Verification items for the finished model (mm, model axes). Face numbers are marked on the shaded views. A direction names the side the tool comes from. Coordinates: 2 decimals unless noted, no trailing zeros. Order: outer loops, then holes, each group sorted by start corner. A loop starts at its lowest first (then second) coordinate and runs counter-clockwise, first axis right, second up. Notation, with made-up numbers: (-12.5, 21) - (3.5, 21) arc R16 cw to (3.5, 52) - close; hole circle Ø11 at (26.5, 64.5). An arc over 180 degrees is marked (long way). One line per question, with ' | ' between items. Start each with the question number.
from build123d import *

# Parameters (mm, degrees)
SKETCH_1_W                = 48.51
SKETCH_1_H                = 34
SKETCH_1_W_2              = 28.51
SKETCH_1_H_2              = 14
EXTRUDE_1_DEPTH           = 12.25
SKETCH_2_R                = 1.91
CUT_EXTRUDE_1_DEPTH       = 33.05257439
SKETCH_4_W                = 13
SKETCH_4_H                = 13.91
EXTRUDE_1_2_DEPTH         = 74.82
SKETCH_5_W                = 13.91
SKETCH_5_H                = 16.23
EXTRUDE_2_DEPTH           = 15
SKETCH_7_R                = 24.5
SKETCH_7_R_2              = 14.5
EXTRUDE_2_2_DEPTH         = 16.23
SKETCH_12_R               = 1.9
CUT_EXTRUDE_4_DEPTH       = 97.312124675
EXTRUDE_3_DEPTH           = 10
EXTRUDE_3_DEPTH_BACK      = 8
SKETCH_13_W               = 13.91
SKETCH_13_H               = 16.23
SKETCH_14_R               = 1.9
CUT_EXTRUDE_5_DEPTH       = 103.744583434
SKETCH_16_W               = 90.709398763
SKETCH_16_H               = 28.955068616
CUT_EXTRUDE_7_DEPTH       = 111.229011154
SKETCH_18_W               = 13
SKETCH_18_H               = 93.080932143
CUT_EXTRUDE_10_DEPTH      = 27
CUT_EXTRUDE_11_DEPTH      = 57
CUT_EXTRUDE_11_DEPTH_BACK = 27
SKETCH_17_W               = 20.23049449
SKETCH_17_H               = 80.723570055


with BuildPart() as part:
    # 草圖1 → Extrude 1 (new body)
    with BuildSketch(Plane(origin=(0, 0, 0), x_dir=(1, 0, 0), z_dir=(0, 1, 0))):
        Rectangle(SKETCH_1_W, SKETCH_1_H)
        Rectangle(SKETCH_1_W_2, SKETCH_1_H_2, mode=Mode.SUBTRACT)
    extrude(amount=EXTRUDE_1_DEPTH)

    # 草圖2 → 除料-伸長1 (cut, through all)
    with BuildSketch(Plane(origin=(0, 12.25, 0), x_dir=(1, 0, 0), z_dir=(0, 1, 0))):
        with Locations(Location((-19.255, 0, 0), (0, 0, 270))):
            Circle(SKETCH_2_R)
        with Locations(Location((19.255, 0, 0), (0, 0, 270))):
            Circle(SKETCH_2_R)
    extrude(amount=-CUT_EXTRUDE_1_DEPTH, mode=Mode.SUBTRACT)

    # 草圖4 → Extrude 1 2 (add)
    with BuildSketch(Plane.XZ):
        with Locations((17.755, 0)):
            Rectangle(SKETCH_4_W, SKETCH_4_H)
    extrude(amount=EXTRUDE_1_2_DEPTH)

    # 草圖5 → Extrude 2 (add)
    with BuildSketch(Plane.ZY.offset(-11.255)):
        with Locations((0, -66.705)):
            Rectangle(SKETCH_5_W, SKETCH_5_H)
    extrude(amount=EXTRUDE_2_DEPTH)

    # 草圖7 → Extrude 2 2 (add)
    with BuildSketch(Plane(origin=(3.626674765, -74.82, 0), x_dir=(1, 0, 0), z_dir=(0, -1, 0))):
        with Locations((-30.978154344, 0)):
            Circle(SKETCH_7_R)
        with Locations((-30.978154344, 0)):
            Circle(SKETCH_7_R_2, mode=Mode.SUBTRACT)
    extrude(amount=-EXTRUDE_2_2_DEPTH)

    # 草圖12 → 除料-伸長4 (cut, through all)
    with BuildSketch(Plane(origin=(0, 0, -6.955), x_dir=(-1, 0, 0), z_dir=(0, 0, -1))):
        with Locations((-3.856713649, -66.705)):
            Circle(SKETCH_12_R)
    extrude(amount=-CUT_EXTRUDE_4_DEPTH, mode=Mode.SUBTRACT)

    # 草圖13 → 填料-伸長3 (add, two sides: drawn at the far end of the back side and taken through both)
    with BuildSketch(Plane(origin=(-55, 0, 0), x_dir=(0, 0, -1), z_dir=(1, 0, 0)).offset(-EXTRUDE_3_DEPTH_BACK)):
        with Locations((0, -66.705)):
            Rectangle(SKETCH_13_W, SKETCH_13_H)
    extrude(amount=EXTRUDE_3_DEPTH + EXTRUDE_3_DEPTH_BACK)

    # 草圖14 → 除料-伸長5 (cut, through all)
    with BuildSketch(Plane(origin=(0, 0, -6.955), x_dir=(-1, 0, 0), z_dir=(0, 0, -1))):
        with Locations((56.908040017, -66.705)):
            Circle(SKETCH_14_R)
    extrude(amount=-CUT_EXTRUDE_5_DEPTH, mode=Mode.SUBTRACT)

    # 草圖16 → 除料-伸長7 (cut, through all)
    with BuildSketch(Plane(origin=(0, 12.25, 0), x_dir=(1, 0, 0), z_dir=(0, 1, 0))):
        with Locations((-17.645300619, -14.477534308)):
            Rectangle(SKETCH_16_W, SKETCH_16_H)
    extrude(amount=-CUT_EXTRUDE_7_DEPTH, mode=Mode.SUBTRACT)

    # 草圖18 → 除料-伸長10 (cut)
    with BuildSketch(Plane.XY):
        with Locations((17.755, -28.279533929)):
            Rectangle(SKETCH_18_W, SKETCH_18_H)
    extrude(amount=-CUT_EXTRUDE_10_DEPTH, mode=Mode.SUBTRACT)


with BuildPart() as cut_extrude_10_piece_1:
    # of the separate pieces the step leaves, piece 1, a body of its own (cut_extrude_10_pieces)
    add(part.part.solids().sort_by_distance((11.255, -58.59, -6.955))[0])


with BuildPart() as cut_extrude_10_piece_2:
    # of the separate pieces the step leaves, piece 2, a body of its own (cut_extrude_10_pieces)
    add(part.part.solids().sort_by_distance((-17.345, 0, 0))[0])

    # 草圖17 → 除料-伸長11 (cut, two sides: drawn at the far end of the back side and taken through both)
    with BuildSketch(Plane.ZY.offset(-11.255).offset(-CUT_EXTRUDE_11_DEPTH_BACK)):
        with Locations((-10.115247245, -18.228214973)):
            Rectangle(SKETCH_17_W, SKETCH_17_H)
    extrude(amount=CUT_EXTRUDE_11_DEPTH + CUT_EXTRUDE_11_DEPTH_BACK, mode=Mode.SUBTRACT)


solid = cut_extrude_10_piece_1.part
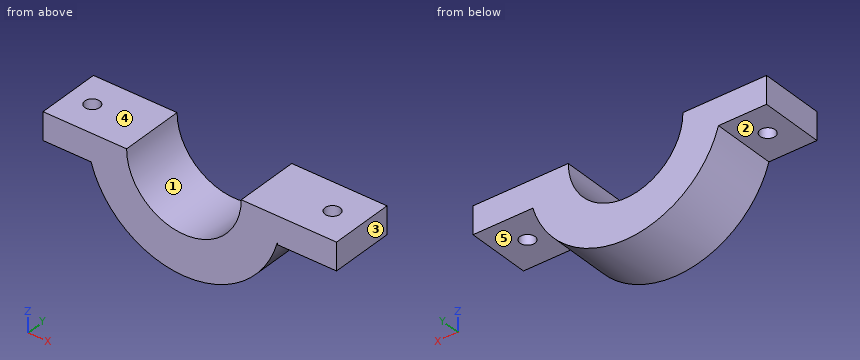
Item 1: Set-up check for the marked faces 4 and 5: record each of +Z, -Z, +X, -X, +Y, -Y from which the full face is reachable in a straight line by a thin tool's end or side.
Item 2: Mould release check, pull along X, two halves, no side actions. Record for the marked faces 1, 2 and 3: +X half, -X half, draft (parallel to the pull), parting line (faces both ways), or undercut.
Item 3: Section check B-B (x = 3). Record the cut outline in (y, z) (3 decimals), then the cut area to 3 significant figures.
Item 4: Section check A-A (z = -2.25). Record the cut outline in (x, y) (3 decimals), then the cut area to 3 significant figures.
Item 5: Section check C-C (z = -10.5). Record the cut outline in (x, y), then the cut area to 3 significant figures.
Item 6: Thickness scan on probe 1 along X at (y, z) = (-65.75, -12.25); probe 2 along Z at (x, y) = (7.5, -73) (3 decimals); probe 3 along X at (y, z) = (-71, -10.25). Record the ranges inside material, lowest first. Write a range as from..to.
Item 7: Section check D-D (y = -70.25). Record the cut outline in (x, z) (3 decimals), then the cut area to 3 significant figures.
Item 8: Gauge pin test, flat ends, axial feed: pin 1 (6 mm diameter, centred on x = -29.5, y = -73, fed in from +Z); pin 2 (4 mm diameter, centred on x = 1, y = -66.5, fed in from -Z) (3 decimals); pin 3 (2.5 mm diameter, centred on x = 3.86, y = -66.7, fed in from -Z); pin 4 (8 mm diameter, centred on y = -73, z = -18.5, fed in from -X). Record the tip position at first contact, or that the pin passes through.
Completed:
1) face 4: +Z, +X, -X, +Y, -Y | face 5: -Z, +X, +Y, -Y
2) face 1: undercut | face 2: draft | face 3: +X half
3) outline: (-74.82, -6.955) - (-68.401, -6.955) - (-68.401, 0) - (-74.82, 0) - close; (-65.009, -6.955) - (-58.59, -6.955) - (-58.59, 0) - (-65.009, 0) - close | area: 89.3 mm^2
4) outline: (-63, -74.82) - (-41.676, -74.82) - (-41.676, -58.59) - (-63, -58.59) - close; (-13.027, -74.82) - (11.255, -74.82) - (11.255, -58.59) - (-13.027, -58.59) - close; hole circle Ø3.8 at (-56.908, -66.705); hole circle Ø3.8 at (3.857, -66.705) | area: 718 mm^2
5) outline: (-49.49, -74.82) - (-37.35, -74.82) - (-37.35, -58.59) - (-49.49, -58.59) - close; (-17.35, -74.82) - (-5.22, -74.82) - (-5.22, -58.59) - (-17.35, -58.59) - close | area: 394 mm^2
6) probe 1: x = -48.57..-35.11, -19.59..-6.13 | probe 2: z = -6.955..0 | probe 3: x = -49.6..-37.61, -17.1..-5.1
7) outline: (-63, -6.955) - (-50.844, -6.955) arc R24.5 ccw to (-3.745, -6.556) - (-3.745, -6.955) - (11.255, -6.955) - (11.255, 0) - (-12.851, 0) arc R14.5 cw to (-41.851, 0) - (-63, 0) - close | area: 793 mm^2
8) pin 1: stops at z = -13.56 | pin 2: stops at z = -6.955 | pin 3: passes through | pin 4: stops at x = -47.1
